The listing builds one solid part. Answer for the finished solid, in the listing's coordinates (mm). Give positions to 0.01 mm unless a question says otherwise; leave off trailing zeros. Write each loop counter-clockwise with the first axis right and the second up, starting at its lowest first coordinate (ties: lowest second). Pieces come first, ordered by that corner, then holes. Notation, with made-up numbers: (89, 67.5) - (100, 67.5) arc R17 ccw to (100, 75.5) - close; hole circle Ø1 at (-12, 41). An arc over 180 degrees is marked (long way). Answer as CSV lines item,"result". Start each with the question number.
(1) Find section C-C (x = 5). Write down the section's boundary in (y, z).
(2) Straight lines are drawn through the part: probe 1 along Z at (x, y) = (19, 2); probe 2 along X at (y, z) = (2.25, -9.5); probe 3 along X at (y, z) = (5.5, 0). For each, find the intervals that lie inside material, in ascending order.
(3) Find section A-A (z = 9.5). Write down the section's boundary in (x, y).
(4) Each of these flat-tipped pins is pushed along its axis until it touches: pin 1 Ø2.5 at (x, z) = (18.86, -9.96) entering from +Y; pin 2 Ø1 at (x, y) = (-18, 6) entering from -Z; pin 3 Ø1 at (x, y) = (17.5, 6) entering from +Z. Where does it stop, or does it pass through?
(5) Find section B-B (z = 1.25). Write down the section's boundary in (x, y), then the cut area to 3 significant figures.
from build123d import *

# Parameters (mm, degrees)
SKETCH1_W               = 41.7195
SKETCH1_H               = 23.9141
BOSS_EXTRUDE1_DEPTH     = 5.2451
CUT_EXTRUDE1_DEPTH      = 25.609170827
CUT_EXTRUDE1_DEPTH_BACK = 25.609170827
SKETCH2_R               = 1
SKETCH3_W               = 4.472619139
SKETCH3_H               = 15.621
SKETCH3_W_2             = 5.720722195
SKETCH3_H_2             = 14.8844
BOSS_EXTRUDE2_DEPTH     = 1.27


with BuildPart() as part:
    # Sketch1 → Boss-Extrude1 (new body)
    with BuildSketch(Plane(origin=(0, 0, 0), x_dir=(1, 0, 0), z_dir=(0, 1, 0))):
        Rectangle(SKETCH1_W, SKETCH1_H)
    extrude(amount=BOSS_EXTRUDE1_DEPTH)

    # Sketch2 → Cut-Extrude1 (cut, two sides: drawn at the far end of the back side and taken through both)
    with BuildSketch(Plane(origin=(0, 5.2451, 0), x_dir=(1, 0, 0), z_dir=(0, 1, 0)).offset(-CUT_EXTRUDE1_DEPTH_BACK)):
        with Locations(Location((-18.85975, 9.95705, 0), (0, 0, 270))):
            Circle(SKETCH2_R)
        with Locations(Location((18.85975, 9.95705, 0), (0, 0, 270))):
            Circle(SKETCH2_R)
        with Locations(Location((18.85975, -9.95705, 0), (0, 0, 270))):
            Circle(SKETCH2_R)
        with Locations(Location((-18.85975, -9.95705, 0), (0, 0, 270))):
            Circle(SKETCH2_R)
    extrude(amount=CUT_EXTRUDE1_DEPTH + CUT_EXTRUDE1_DEPTH_BACK, mode=Mode.SUBTRACT)

    # Sketch3 → Boss-Extrude2 (add)
    with BuildSketch(Plane(origin=(0, 5.2451, 0), x_dir=(1, 0, 0), z_dir=(0, 1, 0))):
        with Locations((18.623440431, 0)):
            Rectangle(SKETCH3_W, SKETCH3_H)
        with Locations((-17.999388903, 0)):
            Rectangle(SKETCH3_W_2, SKETCH3_H_2)
    extrude(amount=BOSS_EXTRUDE2_DEPTH)


solid = part.part
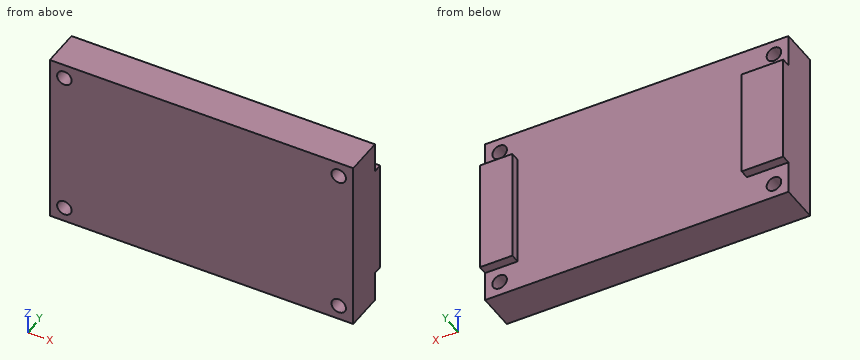
Result set:
1,outline,"(0, -11.96) - (5.25, -11.96) - (5.25, 11.96) - (0, 11.96) - close"
2,probe 1,"-11.96 to -10.95, -8.97 to 8.97, 10.95 to 11.96"
2,probe 2,"-20.86 to -19.75, -17.97 to 17.97, 19.75 to 20.86"
2,probe 3,"-20.86 to -15.14, 16.39 to 20.86"
3,outline,"(-20.86, 0) - (-19.75, 0) - (-19.75, 5.25) - (-20.86, 5.25) - close; (-17.97, 0) - (17.97, 0) - (17.97, 5.25) - (-17.97, 5.25) - close; (19.75, 0) - (20.86, 0) - (20.86, 5.25) - (19.75, 5.25) - close"
4,pin 1,"y = 5.25"
4,pin 2,"z = -7.44"
4,pin 3,"z = 7.81"
5,outline,"(-20.86, 0) - (20.86, 0) - (20.86, 6.52) - (16.39, 6.52) - (16.39, 5.25) - (-15.14, 5.25) - (-15.14, 6.52) - (-20.86, 6.52) - close"
5,area,"232 mm^2"
